Source: CAD feature listing. Evaluate the final solid. Frame: model axes, mm. Face numbers are marked on the shaded views. Coordinates: 2 decimals unless noted, no trailing zeros. Write each loop counter-clockwise with the first axis right and the second up, starting at its lowest first coordinate (ties: lowest second). Pieces come first, ordered by that corner, then holes. Notation, with made-up numbers: M -3.75,25.25 L 52.25,25.25 A19 cw 52.25,52.25 Z; hole C -33.5,89.25 d1. An arc over 180 degrees is marked long. Write item = value, one per line. Start each with the question number.
1. Line query: line 1 along Y through (x, z) = (-70.5, 37); line 2 along Y through (x, z) = (-77.5, 50); line 3 along X through (y, z) = (-61.5, 16). Output: solid intervals per line, ascending.
2. Pin query (flat end, axial travel): pin 1 Ø4 at (x, z) = (-74, 33) entering from +Y; pin 2 Ø10 at (y, z) = (-1.5, 39.5) entering from +X; pin 3 Ø24 at (y, z) = (12.5, 51) entering from -X. Return the tip coordinate at first contact, or that it passes through.
3. Section query A-A (z = 11). Output: boundary loops of the cut face in (x, y), then the cut area to 3 significant figures.
4. Pull-direction query (X, two-part tool) for the marked faces 1, 2, 3 and 4; classes: pulls with the +X half, pulls with the -X half, needs draft (parallel to the pull), parting line crosses it, or undercut.
5. Section query D-D (z = 52). Output: boundary loops of the cut face in (x, y), then the cut area to 3 significant figures.
6. Section query B-B (y = -28). Output: boundary loops of the cut face in (x, z).
7. Section query C-C (x = 22). Output: boundary loops of the cut face in (y, z).
```python
from build123d import *

# Parameters (mm, degrees)
F0_W     = 101.6
F0_H     = 101.6
F1_DEPTH = 76.2
F3_DEPTH = 101.6
F4_W     = 63.5649934411
F4_H     = 88.8701714575
F5_DEPTH = 7.62
F7_DEPTH = 25.4
F8_W     = 7.62
F8_H     = 5.08
F9_DEPTH = 76.2


# Not quite as in the source:
# - a feature names something its author has since deleted; it is built from what else it names


with BuildPart() as f1:
    # F0 (on Top) → F1 (new body)
    with BuildSketch(Plane.XY):
        with Locations((-18.5535050273, 1.2484980512)):
            Rectangle(F0_W, F0_H)
    extrude(amount=F1_DEPTH)

    # F2 (on face) → F3 (cut)
    with BuildSketch(Plane.XZ.offset(49.5515019488)):
        with BuildLine():
            Line((32.2464949727, 76.2), (-50.8901812136, 76.2))
            ThreePointArc((-50.8901812136, 76.2), (-21.4414456403, 24.8771198137), (32.2464949727, 0))
            Line((32.2464949727, 0), (32.2464949727, 76.2))
        make_face()
    extrude(amount=-F3_DEPTH, mode=Mode.SUBTRACT)

    # F4 (on face) → F5 (join)
    with BuildSketch(Plane(origin=(0, 0, 0), x_dir=(1, 0, 0), z_dir=(0, 0, -1))):
        with Locations((-31.7824967206, -2.1479185671)):
            Rectangle(F4_W, F4_H)
    extrude(amount=-F5_DEPTH)

    # F6 (on face) → F7 (join)
    with BuildSketch(Plane.XZ.offset(49.5515019488)):
        with BuildLine():
            Line((-69.3535050273, 76.2), (-69.3535050273, 0))
            Line((-69.3535050273, 0), (32.2464949727, 0))
            ThreePointArc((32.2464949727, 0), (-21.4414456403, 24.8771198137), (-50.8901812136, 76.2))
            Line((-50.8901812136, 76.2), (-69.3535050273, 76.2))
        make_face()
    extrude(amount=F7_DEPTH)

    # F8 (on face) → F9 (join)
    with BuildSketch(Plane(origin=(0, 0, 0), x_dir=(1, 0, 0), z_dir=(0, 0, -1))):
        with BuildLine():
            Line((-76.9735050273, -44.4284980512), (-76.9735050273, -39.3484980512))
            ThreePointArc((-76.9735050273, -39.3484980512), (-86.4529140785, -41.8884980512), (-76.9735050273, -44.4284980512))
        make_face()
        with Locations((-73.1635050273, -41.8884980512)):
            Rectangle(F8_W, F8_H)
        with BuildLine():
            Line((-76.9735050273, 8.9115019488), (-76.9735050273, 13.9915019488))
            ThreePointArc((-76.9735050273, 13.9915019488), (-86.4529140785, 11.4515019488), (-76.9735050273, 8.9115019488))
        make_face()
        with Locations((-73.1635050273, 11.4515019488)):
            Rectangle(F8_W, F8_H)
        with Locations((-73.1635050273, 64.7915019488)):
            Rectangle(F8_W, F8_H)
        with BuildLine():
            ThreePointArc((-76.9735050273, 67.3315019488), (-86.4529140785, 64.7915019488), (-76.9735050273, 62.2515019488))
            Line((-76.9735050273, 62.2515019488), (-76.9735050273, 67.3315019488))
        make_face()
    extrude(amount=-F9_DEPTH)


solid = f1.part
```
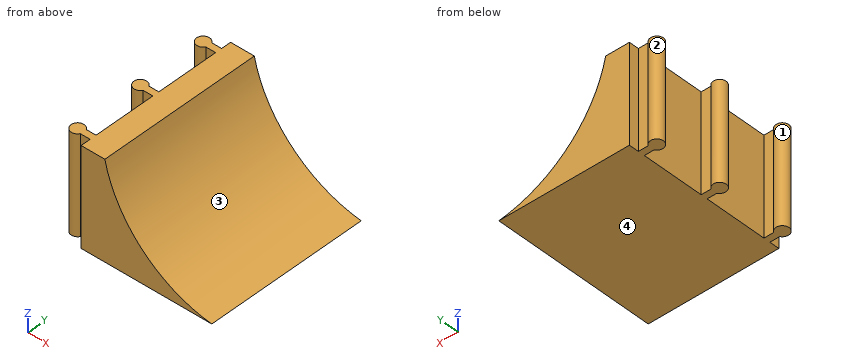
Results are:
q1.line_1 = -67.33 to -62.25, -13.99 to -8.91, 39.35 to 44.43
q1.line_2 = -68.08 to -61.5, -14.74 to -8.16, 38.6 to 45.18
q1.line_3 = -85.24 to -77.5, -69.35 to -10.2
q2.pin_1 = 44.43
q2.pin_2 = -30.6
q2.pin_3 = -69.35
q3.outline = M -76.97,-67.33 L -69.35,-67.33 L -69.35,-74.95 L -1.96,-74.95 L -1.96,52.05 L -69.35,52.05 L -69.35,44.43 L -76.97,44.43 A5.08 ccw long -76.97,39.35 L -69.35,39.35 L -69.35,-8.91 L -76.97,-8.91 A5.08 ccw long -76.97,-13.99 L -69.35,-13.99 L -69.35,-62.25 L -76.97,-62.25 A5.08 ccw long Z
q3.area = 8,910 mm^2
q4.face_1 = undercut
q4.face_2 = undercut
q4.face_3 = pulls with the +X half
q4.face_4 = needs draft
q5.outline = M -76.97,-67.33 L -69.35,-67.33 L -69.35,-74.95 L -42.19,-74.95 L -42.19,52.05 L -69.35,52.05 L -69.35,44.43 L -76.97,44.43 A5.08 ccw long -76.97,39.35 L -69.35,39.35 L -69.35,-8.91 L -76.97,-8.91 A5.08 ccw long -76.97,-13.99 L -69.35,-13.99 L -69.35,-62.25 L -76.97,-62.25 A5.08 ccw long Z
q5.area = 3,800 mm^2
q6.outline = M -69.35,0 L 32.25,0 A97.6 cw -50.89,76.2 L -69.35,76.2 Z
q7.outline = M -74.95,0 L 52.05,0 L 52.05,1.86 L -74.95,1.86 Z
